from build123d import *

# Parameters (mm, degrees)
SKETCH2_W           = 16
SKETCH2_H           = 6
SKETCH2_R           = 2.75
BOSS_EXTRUDE1_DEPTH = 6
SKETCH4_R           = 2.75
SKETCH4_W           = 16
SKETCH4_H           = 6
BOSS_EXTRUDE2_DEPTH = 6


with BuildPart() as part:
    # Sketch2 → Boss-Extrude1 (new body)
    with BuildSketch(Plane.XY):
        with BuildLine():
            ThreePointArc((-14.014958559, -48.70381072), (-7.820513245, -50.092784824), (-1.5, -50.685671098))
            Line((-1.5, -50.685671098), (-1.5, -45.708176163))
            Line((-1.5, -45.708176163), (1.5, -45.708176163))
            Line((1.5, -45.708176163), (1.5, -50.685671098))
            ThreePointArc((1.5, -50.685671098), (7.821643905, -50.09260576), (14.017156267, -48.703168924))
            Line((14.017156267, -48.703168924), (12.476730902, -43.962227135))
            Line((12.476730902, -43.962227135), (15.32990045, -43.035176152))
            Line((15.32990045, -43.035176152), (16.870328795, -47.776127109))
            ThreePointArc((16.870328795, -47.776127109), (22.700337229, -45.258088505), (28.164148211, -42.021379325))
            Line((28.164148211, -42.021379325), (25.229863981, -37.982683562))
            Line((25.229863981, -37.982683562), (27.656914964, -36.219327805))
            Line((27.656914964, -36.219327805), (30.591129228, -40.257927268))
            ThreePointArc((30.591129228, -40.257927268), (35.358240772, -36.060613271), (39.55477218, -31.292812793))
            Line((39.55477218, -31.292812793), (35.511033717, -28.354864828))
            Line((35.511033717, -28.354864828), (37.274389474, -25.927813845))
            Line((37.274389474, -25.927813845), (41.317825829, -28.865542317))
            ThreePointArc((41.317825829, -28.865542317), (44.554494815, -23.399517942), (47.071992795, -17.567224011))
            Line((47.071992795, -17.567224011), (42.313847582, -16.021208913))
            Line((42.313847582, -16.021208913), (43.240898565, -13.168039364))
            Line((43.240898565, -13.168039364), (47.998350807, -14.713829302))
            ThreePointArc((47.998350807, -14.713829302), (49.386863483, -8.514437454), (49.978066205, -2.189019992))
            Line((49.978066205, -2.189019992), (44.972398757, -2.189019992))
            Line((44.972398757, -2.189019992), (44.972398757, 0.810980008))
            Line((44.972398757, 0.810980008), (49.976916317, 0.810980008))
            ThreePointArc((49.976916317, 0.810980008), (49.380832331, 7.136146516), (47.987483994, 13.334664716))
            Line((47.987483994, 13.334664716), (43.22644973, 11.787710909))
            Line((43.22644973, 11.787710909), (42.299398746, 14.640880458))
            Line((42.299398746, 14.640880458), (47.058915168, 16.187341088))
            ThreePointArc((47.058915168, 16.187341088), (44.536626084, 22.0182168), (41.295318935, 27.482188044))
            Line((41.295318935, 27.482188044), (37.246906156, 24.540843989))
            Line((37.246906156, 24.540843989), (35.483550399, 26.967894972))
            Line((35.483550399, 26.967894972), (39.530326401, 29.908049839))
            ThreePointArc((39.530326401, 29.908049839), (35.329326435, 34.673156396), (30.558045552, 38.86714256))
            Line((30.558045552, 38.86714256), (27.619087422, 34.822013725))
            Line((27.619087422, 34.822013725), (25.192036439, 36.585369482))
            Line((25.192036439, 36.585369482), (28.129589934, 40.628565002))
            ThreePointArc((28.129589934, 40.628565002), (22.66202489, 43.861237429), (16.828745179, 46.374658668))
            Line((16.828745179, 46.374658668), (15.285431508, 41.62482759))
            Line((15.285431508, 41.62482759), (12.432261959, 42.551878573))
            Line((12.432261959, 42.551878573), (13.974753738, 47.299180128))
            ThreePointArc((13.974753738, 47.299180128), (7.776727495, 48.683346485), (1.453242586, 49.270700235))
            Line((1.453242586, 49.270700235), (1.453242586, 44.283378765))
            Line((1.453242586, 44.283378765), (-1.546757414, 44.283378765))
            Line((-1.546757414, 44.283378765), (-1.546757414, 49.2608737))
            ThreePointArc((-1.546757414, 49.2608737), (-7.866904098, 48.661958763), (-14.060191394, 47.266915506))
            Line((-14.060191394, 47.266915506), (-12.523488315, 42.537429737))
            Line((-12.523488315, 42.537429737), (-15.376657864, 41.610378754))
            Line((-15.376657864, 41.610378754), (-16.914659767, 46.343861891))
            ThreePointArc((-16.914659767, 46.343861891), (-22.740383136, 43.821308169), (-28.199510335, 40.580897657))
            Line((-28.199510335, 40.580897657), (-25.276621395, 36.557886164))
            Line((-25.276621395, 36.557886164), (-27.703672378, 34.794530407))
            Line((-27.703672378, 34.794530407), (-30.624981542, 38.815367524))
            ThreePointArc((-30.624981542, 38.815367524), (-35.385501758, 34.616974444), (-39.575762572, 29.849294558))
            Line((-39.575762572, 29.849294558), (-35.557791131, 26.93006743))
            Line((-35.557791131, 26.93006743), (-37.321146887, 24.503016447))
            Line((-37.321146887, 24.503016447), (-41.33714976, 27.420813327))
            ThreePointArc((-41.33714976, 27.420813327), (-44.567381262, 21.957845266), (-47.079571363, 16.129696634))
            Line((-47.079571363, 16.129696634), (-42.360604995, 14.596411515))
            Line((-42.360604995, 14.596411515), (-43.287655979, 11.743241967))
            Line((-43.287655979, 11.743241967), (-48.004645978, 13.275884924))
            ThreePointArc((-48.004645978, 13.275884924), (-49.389276358, 7.082804571), (-49.978315717, 0.764222594))
            Line((-49.978315717, 0.764222594), (-45.01915617, 0.764222594))
            Line((-45.01915617, 0.764222594), (-45.01915617, -2.235777406))
            Line((-45.01915617, -2.235777406), (-49.976658896, -2.235777406))
            ThreePointArc((-49.976658896, -2.235777406), (-49.380673152, -8.553500826), (-47.989286669, -14.744855434))
            Line((-47.989286669, -14.744855434), (-43.273207143, -13.212508307))
            Line((-43.273207143, -13.212508307), (-42.34615616, -16.065677856))
            Line((-42.34615616, -16.065677856), (-47.06108419, -17.597650839))
            ThreePointArc((-47.06108419, -17.597650839), (-44.542778803, -23.422507686), (-41.306963736, -28.881474636))
            Line((-41.306963736, -28.881474636), (-37.293663569, -25.965641387))
            Line((-37.293663569, -25.965641387), (-35.530307812, -28.39269237))
            Line((-35.530307812, -28.39269237), (-39.542974081, -31.308065065))
            ThreePointArc((-39.542974081, -31.308065065), (-35.348264075, -36.07058879), (-30.584062086, -40.263392586))
            Line((-30.584062086, -40.263392586), (-27.665844836, -36.246811123))
            Line((-27.665844836, -36.246811123), (-25.238793853, -38.01016688))
            Line((-25.238793853, -38.01016688), (-28.156765996, -42.026410983))
            ThreePointArc((-28.156765996, -42.026410983), (-22.695337069, -45.260635975), (-16.868173537, -47.776899552))
            Line((-16.868173537, -47.776899552), (-15.332188921, -43.049624988))
            Line((-15.332188921, -43.049624988), (-12.479019372, -43.976675971))
            Line((-12.479019372, -43.976675971), (-14.014958559, -48.70381072))
        make_face()
        with Locations((0, -31.708176163)):
            Rectangle(SKETCH2_W, SKETCH2_H, mode=Mode.SUBTRACT)
        with Locations((-17.5, -8.708176163)):
            Circle(SKETCH2_R, mode=Mode.SUBTRACT)
        with Locations((17.5, -8.708176163)):
            Circle(SKETCH2_R, mode=Mode.SUBTRACT)
    extrude(amount=BOSS_EXTRUDE1_DEPTH)

    # Sketch4 → Boss-Extrude2 (add)
    with BuildSketch(Plane(origin=(0, 0, 0), x_dir=(-1, 0, 0), z_dir=(0, 0, -1))):
        with Locations((17.5, -8.708176163)):
            Circle(SKETCH4_R)
        with Locations((-17.5, -8.708176163)):
            Circle(SKETCH4_R)
        with Locations((0, -31.708176163)):
            Rectangle(SKETCH4_W, SKETCH4_H)
    extrude(amount=-BOSS_EXTRUDE2_DEPTH)


solid = part.part
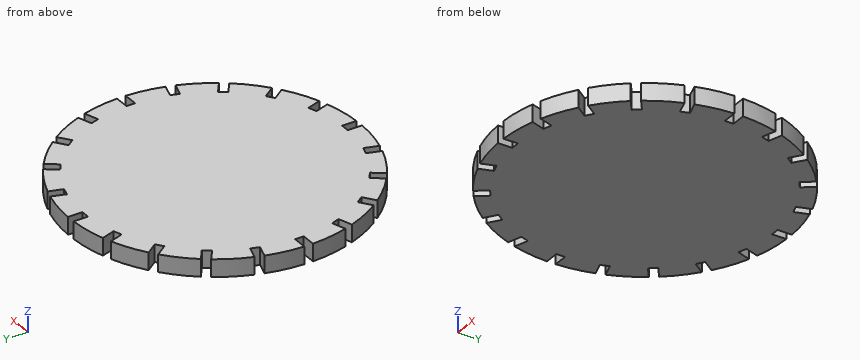
For this review, take the finished solid that the model builds, in its own axes (mm). Coordinates: 2 decimals unless noted, no trailing zeros. Order: outer loops, then holes, each group sorted by start corner. A loop starts at its lowest first (then second) coordinate and runs counter-clockwise, first axis right, second up. Notation, with made-up numbers: (51.25, -39) - (84.25, -39) arc R20 ccw to (84.25, -26) - close; hole circle Ø3 at (0, -39.5). An arc over 180 degrees is marked (long way). Answer as CSV lines item,"result". Start each with the question number.
1) Add section B-B (x = -21). State the section outline as (y, z) points.
2) To check wall thickness, follow line 1 along Y through (x, z) = (44.5, 1.05); line 2 along Y through (x, z) = (-27, 3.75); line 3 along X through (y, z) = (26, 1.85). State the ranges of each line that lie inside material, in increasing order. Write a range as [from, to].
3) Add section A-A (y = -35). State the section outline as (x, z) points.
4) Insertion check: P1, Ø1.5, axis at x = 48, z = 3, coming from the -Y side; P2, Ø1.5, axis at y = -1, z = 2, coming from the +X side; P3, Ø3.5, axis at x = -0.5, z = 3.5, coming from the +Y side. Each pin has a flat end and moves straight along its axis. Give the tip position at first contact, or say it passes through.
Result:
1,outline,"(-46.08, 0) - (44.67, 0) - (44.67, 6) - (-46.08, 6) - close"
2,line 1,"[-23.51, -16.73], [-13.58, 12.2], [15.36, 22.09]"
2,line 2,"[-42.79, -40.43], [-36.73, 35.31], [38.93, 41.38]"
2,line 3,"[-42.27, -39.38], [-36.23, 36.19], [39.26, 42.27]"
3,outline,"(-36.39, 0) - (36.39, 0) - (36.39, 6) - (-36.39, 6) - close"
4,P1,"y = -14.71"
4,P2,"x = 44.97"
4,P3,"y = 49.26"
